Input: dimensioned drawing with shaded views. Units: mm. Origin: part minimum x, y, z. Give positions to 0.01 mm unless a question says otherwise; leave off trailing zeros. Loops run counter-clockwise (first coordinate to the right, second up) from the corner with the lowest first, then second, coordinate; pieces in that order, holes last.
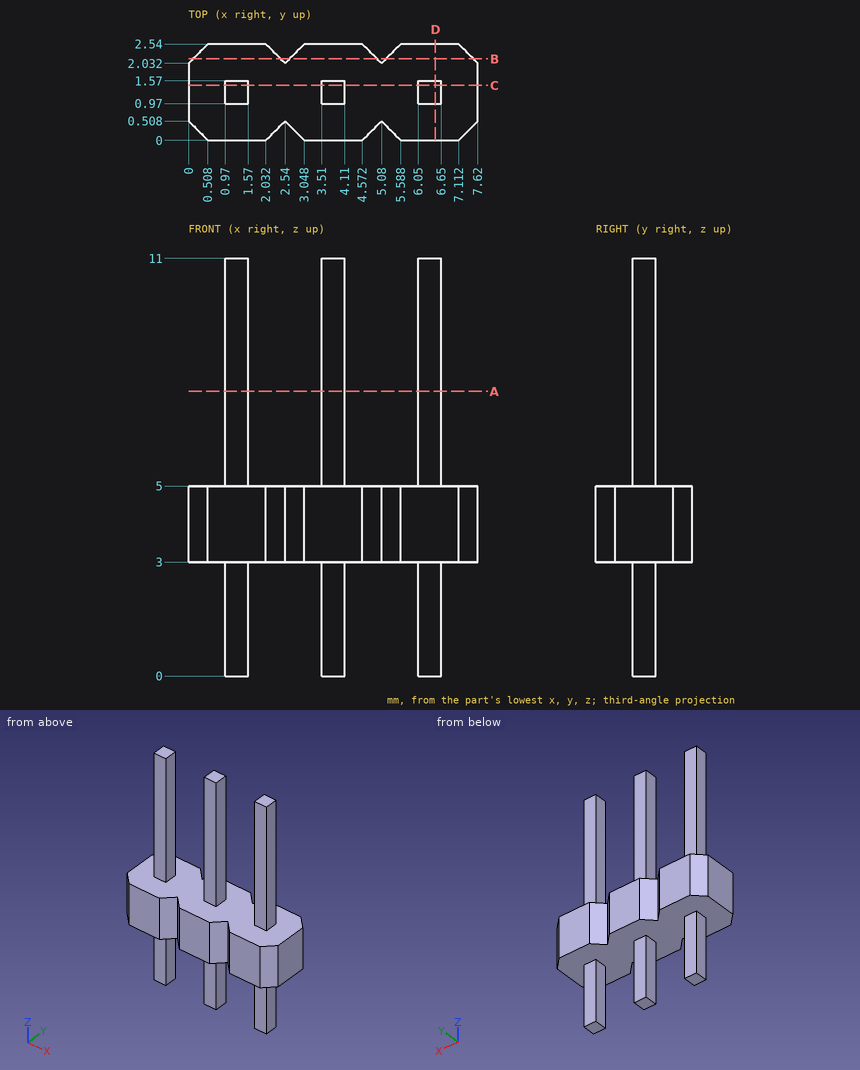
(1) Section A-A, the plane z = 7.5. Return the cut outline in (x, y).
A:
outline: (0.97, 0.97) - (1.57, 0.97) - (1.57, 1.57) - (0.97, 1.57) - close; (3.51, 0.97) - (4.11, 0.97) - (4.11, 1.57) - (3.51, 1.57) - close; (6.05, 0.97) - (6.65, 0.97) - (6.65, 1.57) - (6.05, 1.57) - close
(2) First-contact query: pin 1 (0.5 mm diameter, centred on y = 1.5, z = 1.5, fed in from -X); pin 2 (0.5 mm diameter, centred on y = 1, z = 9, fed in from +X); pin 3 (0.7 mm diameter, centred on x = 6.5, z = 1, fed in from +Y). Flat tips, straight axial feed; report the tip coordinate or a pass-through.
A:
pin 1: stops at x = 0.97
pin 2: stops at x = 6.65
pin 3: stops at y = 1.57
(3) Ray query, line 1 along X through (y, z) = (1.45, 0.5); line 2 along X through (y, z) = (2.2, 4.5); line 3 along Z through (x, y) = (0.75, 0.75). Return the intervals inside material, ascending.
A:
line 1: x = 0.97 to 1.57, 3.51 to 4.11, 6.05 to 6.65
line 2: x = 0.17 to 2.37, 2.71 to 4.91, 5.25 to 7.45
line 3: z = 3 to 5
(4) Section C-C, the plane y = 1.45. Return the cut outline in (x, z).
A:
outline: (0, 3) - (0.97, 3) - (0.97, 0) - (1.57, 0) - (1.57, 3) - (3.51, 3) - (3.51, 0) - (4.11, 0) - (4.11, 3) - (6.05, 3) - (6.05, 0) - (6.65, 0) - (6.65, 3) - (7.62, 3) - (7.62, 5) - (6.65, 5) - (6.65, 11) - (6.05, 11) - (6.05, 5) - (4.11, 5) - (4.11, 11) - (3.51, 11) - (3.51, 5) - (1.57, 5) - (1.57, 11) - (0.97, 11) - (0.97, 5) - (0, 5) - close
(5) Section B-B, the plane y = 2.15. Return the cut outline in (x, z).
A:
outline: (0.12, 3) - (2.42, 3) - (2.42, 5) - (0.12, 5) - close; (2.66, 3) - (4.96, 3) - (4.96, 5) - (2.66, 5) - close; (5.2, 3) - (7.5, 3) - (7.5, 5) - (5.2, 5) - close
(6) Section D-D, the plane x = 6.5. Return the cut outline in (y, z), then the cut area to 3 significant figures.
A:
outline: (0, 3) - (0.97, 3) - (0.97, 0) - (1.57, 0) - (1.57, 3) - (2.54, 3) - (2.54, 5) - (1.57, 5) - (1.57, 11) - (0.97, 11) - (0.97, 5) - (0, 5) - close
area: 10.5 mm2
